Autodesk Inventor part; units mm, degrees
ref_plane "YZ Plane" through (0, 0, 0) normal (1, 0, 0) x (0, 1, 0)
ref_plane "XZ Plane" through (0, 0, 0) normal (0, 1, 0) x (-1, 0, 0)
ref_plane "XY Plane" through (0, 0, 0) normal (0, 0, 1) x (1, 0, 0)
sketch "Sketch3" plane through (0, 0, 0) normal (0, 0, 1) x (1, 0, 0)
  line L0 (0, 0) -> (10, 0)
  line L1 (0, 0) -> (0, 20)
  line L2 (0, 20) -> (8, 20)
  line L3 (10, 0) -> (10, 5)
  line L4 (10, 5) -> (8, 5)
  line L5 (8, 5) -> (8, 7)
  line L6 (8, 7) -> (10, 9.3965)
  line L7 (10, 9.3965) -> (10, 13.3965)
  line L8 (10, 13.3965) -> (8, 20)
  dimension "d17" = 10
  dimension "d18" = 20
  dimension "d19" = 8
  dimension "d40" = 5
  dimension "d43" = 2
  dimension "d44" = 4
  dimension "d45" = 2
revolve "Revolution1" add sketch "Sketch3" angle 360 about axis through (0, 0, 0) along (0, 1, 0)
sketch "Sketch4" plane through (0, 0, 0) normal (0, 1, 0) x (-1, 0, 0)
  circle A0 centre (0, 0) radius 1.6
  dimension "d27" = 3.2
extrude "Extrusion3" cut sketch "Sketch4" along normal through all
sketch "Sketch5" plane through (0, 20, 0) normal (0, 1, 0) x (1, 0, 0)
  circle A0 centre (0, 0) radius 2.65
  dimension "d30" = 5.3
extrude "Extrusion4" cut sketch "Sketch5" against normal blind 5
sketch "Sketch6" plane through (0, 0, 0) normal (0, -1, 0) x (1, 0, 0)
  circle A0 centre (-6, 0) radius 1.5
  circle A1 centre (6, 0) radius 1.5
  circle A2 centre (0, 0) radius 1.6
  line L0 (-6, 0) -> (0, 0) construction
  line L1 (0, 0) -> (6, 0) construction
  dimension "d33" = 3
  dimension "d35" = 3
  dimension "d47" = 6
extrude "Extrusion5" [suppressed]
equation "\"d35\" = d33"
equation "\"d47\" = 2 * d33"
properties part number "modular-post"
Check sheet for the modelled part. Datum: model origin and axes. Units: mm. A direction names the side the tool comes from. Round coordinates to 2 decimals unless told otherwise and drop trailing zeros. Order: outer loops, then holes, each group sorted by start corner. A loop starts at its lowest first (then second) coordinate and runs counter-clockwise, first axis right, second up. Notation, with made-up numbers: (78.5, -17) - (137.5, -17) arc R24 cw to (137.5, 19) - close; hole circle Ø8 at (53, 60). An arc over 180 degrees is marked (long way). Answer as CSV lines item,"result". Start each with the question number.
1) Section check A-A (x = 0). Record the cut outline in (y, z), then the cut area to 4 significant figures.
2) Depth check by flat-ended pin: pin 1 (1.5 mm diameter, centred on y = 9.5, z = -2, fed in from -X); pin 2 (6 mm diameter, centred on x = -4.5, y = 16.5, fed in from +Z); pin 3 (5 mm diameter, centred on y = 5, z = 5, fed in from +X). Enter the tip coordinate at first touch or a pass-through.
3) Section check B-B (z = 0). Record the cut outline in (x, y), then the cut area to 4 significant figures.
4) Draft check along Y on faces 1 (the face through (-2.17, 2.54, 9.76)), 2 (the face through (-2, 20, -2)), 3 (the face through (-1.76, 7.15, 7.93)). Enter one of: +Y half, -Y half, draft (parallel to the pull), parting line (faces both ways), or undercut.
5) Tool access check on faces 4 (the face through (-1.73, 6.01, 7.81)), 5 (the face through (0, 15, 2)), 6 (the face through (2, 0, 0)). Record the directions out of +Z, -Z, +X, -X, +Y, -Y that give a thin tool (end or side, any length) a straight path to the whole face; none if there is none.
6) Scan lines: probe 1 along Z at (x, y) = (0, 4); probe 2 along X at (y, z) = (5.5, 0). Record each from-to range of solid material in increasing order.
Determined:
1,outline,"(0, -10) - (5, -10) - (5, -8) - (7, -8) - (9.4, -10) - (13.4, -10) - (20, -8) - (20, -2.65) - (15, -2.65) - (15, -1.6) - (0, -1.6) - close; (0, 1.6) - (15, 1.6) - (15, 2.65) - (20, 2.65) - (20, 8) - (13.4, 10) - (9.4, 10) - (7, 8) - (5, 8) - (5, 10) - (0, 10) - close"
1,area,"299.5 mm^2"
2,pin 1,"x = -9.92"
2,pin 2,"z = 9.41"
2,pin 3,"x = 9.68"
3,outline,"(-10, 0) - (-1.6, 0) - (-1.6, 15) - (-2.65, 15) - (-2.65, 20) - (-8, 20) - (-10, 13.4) - (-10, 9.4) - (-8, 7) - (-8, 5) - (-10, 5) - close; (1.6, 0) - (10, 0) - (10, 5) - (8, 5) - (8, 7) - (10, 9.4) - (10, 13.4) - (8, 20) - (2.65, 20) - (2.65, 15) - (1.6, 15) - close"
3,area,"299.5 mm^2"
4,face 1,"draft"
4,face 2,"+Y half"
4,face 3,"undercut"
5,face 4,"none"
5,face 5,"+Y"
5,face 6,"+Z, -Z, +X, -X, -Y"
6,probe 1,"-10 to -1.6, 1.6 to 10"
6,probe 2,"-8 to -1.6, 1.6 to 8"
